```python
from build123d import *

# Parameters (mm, degrees)
F0_W     = 184.15
F0_H     = 53.975
F1_DEPTH = 3.175
F3_D     = 3
F4_W     = 25.4
F4_H     = 25.4
F5_DEPTH = 25.4
F6_W     = 158.75
F6_H     = 3.175
F7_DEPTH = 79.375


with BuildPart() as f1:
    # F0 (on Top) → F1 (new body)
    with BuildSketch(Plane.XY):
        with Locations((-92.075, 26.9875)):
            Rectangle(F0_W, F0_H)
    extrude(amount=F1_DEPTH)

    # F3 (through all)
    with Locations(Plane.XY.offset(3.175)):
        with Locations((-177.8, 47.625), (-6.35, 47.625)):
            Hole(F3_D / 2)

    # F4 (on face) → F5 (cut)
    with BuildSketch(Plane.XY.offset(3.175)):
        with Locations((-12.7, 12.7)):
            Rectangle(F4_W, F4_H)
    extrude(amount=-F5_DEPTH, mode=Mode.SUBTRACT)

    # F6 (on face) → F7 (join)
    with BuildSketch(Plane(origin=(0, 0, 0), x_dir=(1, 0, 0), z_dir=(0, 0, -1))):
        with Locations((-104.775, -1.5875)):
            Rectangle(F6_W, F6_H)
    extrude(amount=F7_DEPTH)


solid = f1.part
```
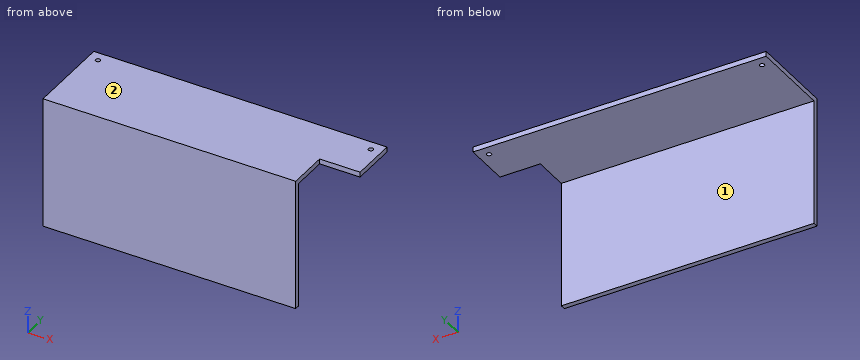
Geometry: final body of the model. Coordinates: model frame, mm. Face numbers are marked on the shaded views. A direction names the side the tool comes from. Coordinates: 2 decimals unless noted, no trailing zeros. Loops run counter-clockwise (first coordinate to the right, second up) from the corner with the lowest first, then second, coordinate; pieces in that order, holes last. Notation, with made-up numbers: (30.5, -7.5) -> (46.5, -7.5) arc R22 cw to (46.5, 25.5) -> close; hole circle Ø11 at (-3, 28.25). An arc over 180 degrees is marked (long way). Use a Markdown table: item, result. Add a question column.
(1) Section query A-A, the plane x = -92.5. Return loops of the section in (y, z) (3 decimals).
(2) Access query for the marked faces 1 and 2. Directions: +Z, -Z, +X, -X, +Y, -Y. A direction counts if a zero-diameter tool reaches every point of the face in a straight line with its end or side. Return the directions, or none.
(3) Pin query (flat end, axial travel): pin 1 Ø12.5 at (y, z) = (6.5, -45) entering from +X; pin 2 Ø1.5 at (x, y) = (-140.5, 47) entering from -Z; pin 3 Ø2.5 at (x, z) = (-11, 2.5) entering from -Y. Return the tip coordinate at first contact, or that it passes through.
(4) Section query B-B, the plane y = 7.5. Return loops of the section in (x, z) (3 decimals), plus the area to 3 significant figures.
(5) Line query: line 1 along Y through (x, z) = (-6.35, 1.8) (3 decimals); line 2 along Y through (x, z) = (-177.8, 1.75) (3 decimals); line 3 along Z through (x, y) = (-158.5, 18) (3 decimals). Output: solid intervals per line, ascending.
Answer:
| question | item | result |
|---|---|---|
| 1 | outline | (0, -79.375) -> (3.175, -79.375) -> (3.175, 0) -> (53.975, 0) -> (53.975, 3.175) -> (0, 3.175) -> close |
| 2 | face 1 | -Z, +X, -X, +Y |
| 2 | face 2 | +Z, +X, -X, +Y, -Y |
| 3 | pin 1 | stops at x = -25.4 |
| 3 | pin 2 | stops at z = 0 |
| 3 | pin 3 | stops at y = 25.4 |
| 4 | outline | (-184.15, 0) -> (-25.4, 0) -> (-25.4, 3.175) -> (-184.15, 3.175) -> close |
| 4 | area | 504 mm^2 |
| 5 | line 1 | y = 25.4 to 46.125, 49.125 to 53.975 |
| 5 | line 2 | y = 0 to 46.125, 49.125 to 53.975 |
| 5 | line 3 | z = 0 to 3.175 |
